```python
from build123d import *

# Parameters (mm, degrees)
F1_DEPTH  = 25.4
F1_FACE_W = 25.4
F1_FACE_H = 3.175
F2_DEPTH  = 50.8
F4_D      = 3.175
F6_D      = 3.175


with BuildPart() as f1:
    # F0 (on Right) → F1 (new body)
    with BuildSketch(Plane.YZ):
        with BuildLine():
            Line((3.175, 0), (0, 0))
            ThreePointArc((0, 0), (53.209829, -91.088205), (152.4, -127))
            Line((152.4, -127), (152.4, -123.825))
            ThreePointArc((152.4, -123.825), (55.44546, -88.837522), (3.175, 0))
        make_face()
        with BuildLine():
            Line((152.4, -123.825), (152.4, -127))
            ThreePointArc((152.4, -127), (251.590171, -91.088205), (304.8, 0))
            Line((304.8, 0), (301.625, 0))
            ThreePointArc((301.625, 0), (249.35454, -88.837522), (152.4, -123.825))
        make_face()
    extrude(amount=F1_DEPTH)

    # F1_face (on face) → F2 (join)
    with BuildSketch(Plane(origin=(12.7, 1.5875, 0), x_dir=(1, 0, 0), z_dir=(0, 0, 1))):
        Rectangle(F1_FACE_W, F1_FACE_H)
        with Locations((0, 301.625)):
            Rectangle(F1_FACE_W, F1_FACE_H)
    extrude(amount=F2_DEPTH)

    # F4 (through all)
    with Locations(Plane(origin=(0, 304.8, 0), x_dir=(-1, 0, 0), z_dir=(0, 1, 0))):
        with Locations((-12.7, 38.1), (-12.7, 12.7)):
            Hole(F4_D / 2)

    # F6 (through all)
    with Locations(Plane.XY):
        with Locations((12.7, 76.2), (12.7, 228.6)):
            Hole(F6_D / 2)


solid = f1.part
```
Could you check a few things on this model? Use its own coordinates, in mm. Give positions to 0.01 mm unless a question says otherwise; leave off trailing zeros. Write each loop counter-clockwise with the first axis right and the second up, starting at its lowest first coordinate (ties: lowest second). Pieces come first, ordered by that corner, then holes. Notation, with made-up numbers: (13.5, 10.5) - (36.5, 10.5) arc R31 ccw to (36.5, 34.5) - close; hole circle Ø3 at (89, 79). An arc over 180 degrees is marked (long way). One line per item, written item: value. Start each with the question number.
Item 1: If we mould it in two halves opening along Y, with no side actions, what happens to faces 1 (the face through (13, 301.625, 25)), 2 (the face through (0, 152, -124)), 3 (the face through (13, 3.175, 25)), 4 (the face through (13, 304.8, 25))? For each: +Y half, -Y half, draft (parallel to the pull), parting line (faces both ways), or undercut.
Item 2: Imagine slicing it at D-D, the plane y = 126. List the corners of the cut face in (x, z) for me, and give its area (3 significant figures).
Item 3: Imagine slicing it at B-B, the plane x = 18. List the corners of the cut face in (y, z) for me (3 decimals).
Item 4: Imagine slicing it at C-C, the plane z = -30.5. List the corners of the cut face in (x, y) for me, and give its area (3 significant figures).
Item 5: Imagine slicing it at A-A, the plane z = 28. List the corners of the cut face in (x, y) for me (3 decimals).
Item 6: I'm going to push flat-ended pins straight in: pin 1 (4 mm diameter, centred on x = 12.7, y = 76.2, fed in from -Z); pin 2 (4 mm diameter, centred on x = 12.5, y = 106, fed in from -Z); pin 3 (5 mm diameter, centred on x = 12.7, z = 38.1, fed in from -Y); pin 4 (10 mm diameter, centred on x = 12, y = 161.5, fed in from -Z). Where does each tip first touch, or does it pass through?
Item 7: Please list where these lines run through material, in increasing order: line 1 (Y direction, x = 7.25, z = 14) (3 decimals); line 2 (Y direction, x = 12.7, z = -105.3); line 3 (X direction, y = 302, z = 38). Write a range as from..to.
Geometry says:
1. face 1: undercut
1. face 2: draft
1. face 3: undercut
1. face 4: +Y half
2. outline: (0, -124.73) - (25.4, -124.73) - (25.4, -121.51) - (0, -121.51) - close
2. area: 81.8 mm^2
3. outline: (0, 0) arc R154.94 ccw to (304.8, 0) - (304.8, 50.8) - (301.625, 50.8) - (301.625, 0) arc R151.83 cw to (152.4, -123.825) arc R151.83 cw to (3.175, 0) - (3.175, 50.8) - (0, 50.8) - close
4. outline: (0, 8.9) - (25.4, 8.9) - (25.4, 12.29) - (0, 12.29) - close; (0, 292.51) - (25.4, 292.51) - (25.4, 295.9) - (0, 295.9) - close
4. area: 172 mm^2
5. outline: (0, 0) - (25.4, 0) - (25.4, 3.175) - (0, 3.175) - close; (0, 301.625) - (25.4, 301.625) - (25.4, 304.8) - (0, 304.8) - close
6. pin 1: z = -108.08
6. pin 2: z = -120.5
6. pin 3: y = 0
6. pin 4: z = -126.95
7. line 1: 0..3.175, 301.625..304.8
7. line 2: 73.32..74.61, 77.79..79.72, 225.08..227.01, 230.19..231.48
7. line 3: 0..11.12, 14.28..25.4
